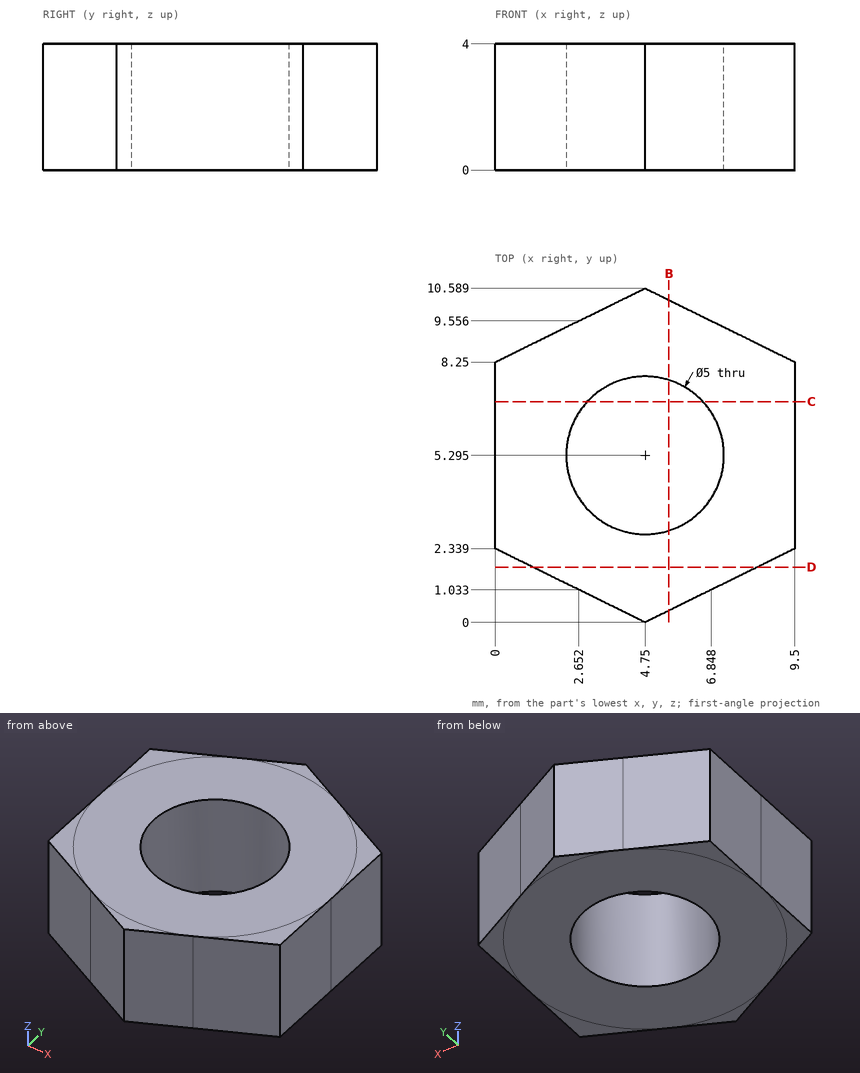
Here's the drawing with two shaded views (mm, measured from the low corner). I have some questions. Round coordinates to 2 decimals unless told otherwise and drop trailing zeros. Write each loop counter-clockwise with the first axis right and the second up, starting at its lowest first coordinate (ties: lowest second). Pieces come first, ordered by that corner, then holes. Notation, with made-up numbers: M 1,17.5 L 53,17.5 A24 cw 53,52.5 Z; hole C 78,44 d9. An arc over 180 degrees is marked long. Write each question's results on one line, items separated by ' | '. Start each with the question number.
1. Imagine slicing it at C-C on y = 7. List the corners of the cut face in (x, z) for me.
2. Imagine slicing it at D-D on y = 1.75. List the corners of the cut face in (x, z) for me (1 decimal).
3. I'm going to push a flat-ended pin straight in: pin 1 Ø1 at (x, z) = (7, 2) entering from -Y. Where does the tip first touch, or does it pass through?
4. I need wall thicknesses on L1, parallel to X at y = 6.25, z = 3.1; L2, parallel to X at y = 3, z = 2.4 (1 decimal); L3, parallel to Y at x = 2.75, z = 2.9 (1 decimal). Which ranges of each line are inside material? Lowest first, please. Write a range as from..to.
5. Imagine slicing it at B-B on x = 5.5. List the corners of the cut face in (y, z) for me, and give its area (3 significant figures).
Result sheet:
1) outline: M 0,0 L 2.92,0 L 2.92,4 L 0,4 Z; M 6.58,0 L 9.5,0 L 9.5,4 L 6.58,4 Z
2) outline: M 1.2,0 L 8.3,0 L 8.3,4 L 1.2,4 Z
3) pin 1: stops at y = 0.86
4) L1: x = 0..2.44, 7.06..9.5 | L2: x = 0..3.8, 5.7..9.5 | L3: y = 1..3.8, 6.8..9.6
5) outline: M 0.37,0 L 2.91,0 L 2.91,4 L 0.37,4 Z; M 7.68,0 L 10.22,0 L 10.22,4 L 7.68,4 Z | area: 20.3 mm^2
